Source: CAD feature listing. Evaluate the final solid. Frame: model axes, mm. Face numbers are marked on the shaded views. Coordinates: 2 decimals unless noted, no trailing zeros. Loops run counter-clockwise (first coordinate to the right, second up) from the corner with the lowest first, then second, coordinate; pieces in that order, holes last.
Item 1: Pin query (flat end, axial travel): pin 1 Ø1.5 at (x, z) = (-3.5, 2.5) entering from -Y; pin 2 Ø0.6 at (x, y) = (2, 1.5) entering from -Z; pin 3 Ø8 at (y, z) = (27, -11) entering from -X; pin 4 Ø1.5 at (x, z) = (-8, -7.5) entering from +Y. Return the tip coordinate at first contact, or that it passes through.
Item 2: Line query: probe 1 along X at (y, z) = (5, -8); probe 2 along Y at (x, z) = (7, 2); probe 3 along Z at (x, y) = (23, 46). Output: solid intervals per line, ascending.
Item 3: Section query D-D, the plane z = -24. Return the cut outline in (x, y).
Item 4: Pull-direction query (X, two-part tool) for the marked faces 1, 2, 3 and 4; classes: +X half, -X half, draft (parallel to the pull), parting line (faces both ways), or undercut.
Item 5: Section query B-B, the plane y = 17.5. Return the cut outline in (x, z), then the cut area to 3 significant figures.
Item 6: Section query C-C, the plane z = 7.5. Return the cut outline in (x, y).
Item 7: Section query A-A, the plane x = 9. Return the cut outline in (y, z).
```python
from build123d import *

# Parameters (mm, degrees)
SKETCH1_W           = 82
SKETCH1_H           = 22
BOSS_EXTRUDE1_DEPTH = 2
EXTRUDE_THIN2_DEPTH = 78
BOSS_EXTRUDE2_DEPTH = 0.5
BOSS_EXTRUDE3_DEPTH = 0.5


with BuildPart() as part:
    # Sketch1 → Boss-Extrude1 (new body)
    with BuildSketch(Plane(origin=(0, 0, 0), x_dir=(1, 0, 0), z_dir=(0, 1, 0))):
        Rectangle(SKETCH1_W, SKETCH1_H)
    extrude(amount=BOSS_EXTRUDE1_DEPTH)

    # Sketch4 → Extrude-Thin2 (add)
    with BuildSketch(Plane(origin=(-39, 0, 0), x_dir=(0, 0, -1), z_dir=(1, 0, 0))):
        Polygon((8.5, 2), (27.911428383, 74.444436972), (28.635872752, 74.250322688), (9.22444437, 1.805885716), align=None)
    extrude(amount=EXTRUDE_THIN2_DEPTH)

    # Sketch5 → Boss-Extrude2 (add)
    with BuildSketch(Plane(origin=(39, 0, 0), x_dir=(0, 0, -1), z_dir=(1, 0, 0))):
        Polygon((-8.5, 2), (1.852761804, 40.637033052), (18.852761804, 40.637033052), (8.5, 2), align=None)
    extrude(amount=-BOSS_EXTRUDE2_DEPTH)

    # Sketch6 → Boss-Extrude3 (add)
    with BuildSketch(Plane(origin=(-39, 0, 0), x_dir=(0, 0, -1), z_dir=(1, 0, 0))):
        Polygon((-8.5, 2), (1.852761804, 40.637033052), (18.852761804, 40.637033052), (8.5, 2), align=None)
    extrude(amount=BOSS_EXTRUDE3_DEPTH)


solid = part.part
```
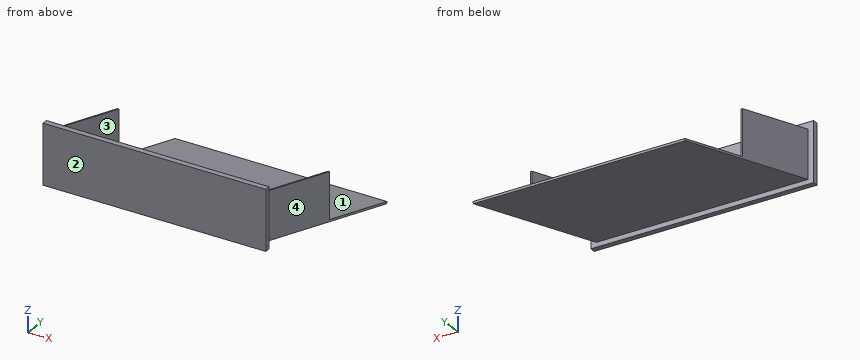
Verdict:
1. pin 1: stops at y = 0
1. pin 2: stops at z = -11
1. pin 3: stops at x = -39
1. pin 4: stops at y = 2
2. probe 1: x = -39 to -38.5, 38.5 to 39
2. probe 2: y = 0 to 2
2. probe 3: z = -21.07 to -20.29
3. outline: (-39, 56.95) - (39, 56.95) - (39, 59.85) - (-39, 59.85) - close
4. face 1: undercut
4. face 2: draft
4. face 3: undercut
4. face 4: +X half
5. outline: (-39, -13.43) - (39, -13.43) - (39, 4.35) - (38.5, 4.35) - (38.5, -12.65) - (-38.5, -12.65) - (-38.5, 4.35) - (-39, 4.35) - close
5. area: 77.6 mm2
6. outline: (-41, 0) - (41, 0) - (41, 2) - (39, 2) - (39, 5.73) - (38.5, 5.73) - (38.5, 2) - (-38.5, 2) - (-38.5, 5.73) - (-39, 5.73) - (-39, 2) - (-41, 2) - close
7. outline: (0, -11) - (2, -11) - (2, -9.28) - (74.25, -28.64) - (74.44, -27.91) - (2, -8.5) - (2, 11) - (0, 11) - close
